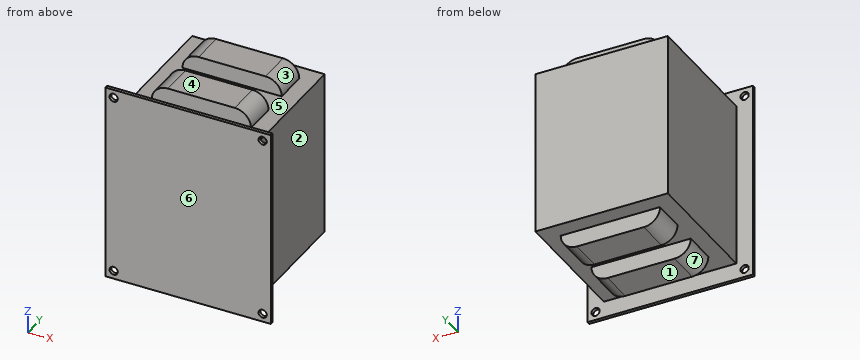
from build123d import *

# Parameters (mm, degrees)
SKETCH1_W           = 127
SKETCH1_H           = 152.4
SKETCH1_R           = 3.175
SKETCH1_W_2         = 101.6
SKETCH1_H_2         = 127
BOSS_EXTRUDE1_DEPTH = 2.54
SKETCH1_4_W         = 101.6
SKETCH1_4_H         = 127
BOSS_EXTRUDE2_DEPTH = 101.6
BOSS_EXTRUDE3_START = 63.5
BOSS_EXTRUDE3_DEPTH = 25.4
BOSS_EXTRUDE4_START = 19.05
BOSS_EXTRUDE4_DEPTH = 25.4


with BuildPart() as part:
    # Sketch1 → Boss-Extrude1 (new body)
    with BuildSketch(Plane(origin=(0, 0, 0), x_dir=(1, 0, 0), z_dir=(0, 1, 0))):
        Rectangle(SKETCH1_W, SKETCH1_H)
        with Locations((-57.15, -69.85)):
            Circle(SKETCH1_R, mode=Mode.SUBTRACT)
        with Locations((57.15, -69.85)):
            Circle(SKETCH1_R, mode=Mode.SUBTRACT)
        with BuildLine():
            Line((-50.8, -63.5), (-50.8, 63.5))
            Line((-50.8, 63.5), (-38.1, 63.5))
            ThreePointArc((-38.1, 63.5), (-34.454650999, 72.300650999), (-25.654, 75.946))
            Line((-25.654, 75.946), (25.654, 75.946))
            ThreePointArc((25.654, 75.946), (34.454650999, 72.300650999), (38.1, 63.5))
            Line((38.1, 63.5), (50.8, 63.5))
            Line((50.8, 63.5), (50.8, -63.5))
            Line((50.8, -63.5), (38.1, -63.5))
            ThreePointArc((38.1, -63.5), (34.454650999, -72.300650999), (25.654, -75.946))
            Line((25.654, -75.946), (-25.654, -75.946))
            ThreePointArc((-25.654, -75.946), (-34.454650999, -72.300650999), (-38.1, -63.5))
            Line((-38.1, -63.5), (-50.8, -63.5))
        make_face(mode=Mode.SUBTRACT)
        with Locations((-57.15, 69.85)):
            Circle(SKETCH1_R, mode=Mode.SUBTRACT)
        with Locations((57.15, 69.85)):
            Circle(SKETCH1_R, mode=Mode.SUBTRACT)
        with BuildLine():
            Line((38.1, -63.5), (-38.1, -63.5))
            ThreePointArc((-38.1, -63.5), (-34.454650999, -72.300650999), (-25.654, -75.946))
            Line((-25.654, -75.946), (25.654, -75.946))
            ThreePointArc((25.654, -75.946), (34.454650999, -72.300650999), (38.1, -63.5))
        make_face()
        Rectangle(SKETCH1_W_2, SKETCH1_H_2)
        with BuildLine():
            ThreePointArc((-25.654, 75.946), (-34.454650999, 72.300650999), (-38.1, 63.5))
            Line((-38.1, 63.5), (38.1, 63.5))
            ThreePointArc((38.1, 63.5), (34.454650999, 72.300650999), (25.654, 75.946))
            Line((25.654, 75.946), (-25.654, 75.946))
        make_face()
    extrude(amount=BOSS_EXTRUDE1_DEPTH)

    # Sketch1<4> → Boss-Extrude2 (add)
    with BuildSketch(Plane(origin=(0, 0, 0), x_dir=(1, 0, 0), z_dir=(0, 1, 0))):
        Rectangle(SKETCH1_4_W, SKETCH1_4_H)
    extrude(amount=BOSS_EXTRUDE2_DEPTH)

    # Sketch1<5> → Boss-Extrude3 (add)
    with BuildSketch(Plane(origin=(0, 0, 0), x_dir=(1, 0, 0), z_dir=(0, 1, 0)).offset(BOSS_EXTRUDE3_START)):
        with BuildLine():
            Line((38.1, -63.5), (-38.1, -63.5))
            ThreePointArc((-38.1, -63.5), (-34.454650999, -72.300650999), (-25.654, -75.946))
            Line((-25.654, -75.946), (25.654, -75.946))
            ThreePointArc((25.654, -75.946), (34.454650999, -72.300650999), (38.1, -63.5))
        make_face()
        with BuildLine():
            Line((25.654, 75.946), (-25.654, 75.946))
            ThreePointArc((-25.654, 75.946), (-34.454650999, 72.300650999), (-38.1, 63.5))
            Line((-38.1, 63.5), (38.1, 63.5))
            ThreePointArc((38.1, 63.5), (34.454650999, 72.300650999), (25.654, 75.946))
        make_face()
    extrude(amount=BOSS_EXTRUDE3_DEPTH)

    # Sketch1<6> → Boss-Extrude4 (add)
    with BuildSketch(Plane(origin=(0, 0, 0), x_dir=(1, 0, 0), z_dir=(0, 1, 0)).offset(BOSS_EXTRUDE4_START)):
        with BuildLine():
            Line((38.1, -63.5), (-38.1, -63.5))
            ThreePointArc((-38.1, -63.5), (-34.454650999, -72.300650999), (-25.654, -75.946))
            Line((-25.654, -75.946), (25.654, -75.946))
            ThreePointArc((25.654, -75.946), (34.454650999, -72.300650999), (38.1, -63.5))
        make_face()
        with BuildLine():
            ThreePointArc((-25.654, 75.946), (-34.454650999, 72.300650999), (-38.1, 63.5))
            Line((-38.1, 63.5), (38.1, 63.5))
            ThreePointArc((38.1, 63.5), (34.454650999, 72.300650999), (25.654, 75.946))
            Line((25.654, 75.946), (-25.654, 75.946))
        make_face()
    extrude(amount=BOSS_EXTRUDE4_DEPTH)


solid = part.part
Model file for the job. Use its own axes, mm. Face numbers are marked on the shaded views. A direction names the side the tool comes from. Give positions to 0.01 mm unless a question says otherwise; leave off trailing zeros. Loops run counter-clockwise (first coordinate to the right, second up) from the corner with the lowest first, then second, coordinate; pieces in that order, holes last.
1) Saw through at A-A (x = 57.15). Write the cut outline in (y, z) (3 decimals).
2) Wall check: line 1 (Z direction, x = 57.15, y = 1.3) (3 decimals); line 2 (X direction, y = 1.45, z = -69.85) (3 decimals); line 3 (Y direction, x = -57.5, z = -58.5). Give the ranges that are in metal, low to high.
3) Saw through at B-B (z = -9.5). Write the cut outline in (x, y).
4) Pull direction Y, two halves, no side cores. Call the marked faces 5, 6 and 7: +Y half, -Y half, draft (parallel to the pull), parting line (faces both ways), or undercut.
5) Saw through at D-D (z = 69.85). Write the cut outline in (x, y) (3 decimals).
6) Flat gauge pins, fed straight in: pin 1 Ø13.5 at (x, z) = (10, -73) entering from +Y; pin 2 Ø8 at (y, z) = (87.5, 54.5) entering from -X; pin 3 Ø1 at (y, z) = (78.5, -4.5) entering from +X; pin 4 Ø5 at (x, z) = (-57.15, -69.85) entering from +Y. Where does each tip first touch, or does it go through?
7) Saw through at C-C (y = 84.5). Write the cut outline in (x, z).
8) Tool access for the marked faces 1, 2, 3 and 4: list every direction of +Z, -Z, +X, -X, +Y, -Y with a clear straight run to the whole face (end or side of a thin tool).
Answer block:
1. outline: (0, -76.2) - (2.54, -76.2) - (2.54, -73.025) - (0, -73.025) - close; (0, -66.675) - (2.54, -66.675) - (2.54, 66.675) - (0, 66.675) - close; (0, 73.025) - (2.54, 73.025) - (2.54, 76.2) - (0, 76.2) - close
2. line 1: z = -76.2 to -73.025, -66.675 to 66.675, 73.025 to 76.2
2. line 2: x = -63.5 to -60.325, -53.975 to 53.975, 60.325 to 63.5
2. line 3: y = 0 to 2.54
3. outline: (-63.5, 0) - (63.5, 0) - (63.5, 2.54) - (50.8, 2.54) - (50.8, 101.6) - (-50.8, 101.6) - (-50.8, 2.54) - (-63.5, 2.54) - close
4. face 5: undercut
4. face 6: -Y half
4. face 7: draft
5. outline: (-63.5, 0) - (-60.325, 0) - (-60.325, 2.54) - (-63.5, 2.54) - close; (-53.975, 0) - (53.975, 0) - (53.975, 2.54) - (-53.975, 2.54) - close; (-36.358, 19.05) - (36.358, 19.05) - (36.358, 44.45) - (-36.358, 44.45) - close; (-36.358, 63.5) - (36.358, 63.5) - (36.358, 88.9) - (-36.358, 88.9) - close; (60.325, 0) - (63.5, 0) - (63.5, 2.54) - (60.325, 2.54) - close
6. pin 1: stops at y = 88.9
6. pin 2: stops at x = -50.8
6. pin 3: stops at x = 50.8
6. pin 4: passes through
7. outline: (-50.8, -63.5) - (-38.1, -63.5) arc R12.45 ccw to (-25.65, -75.95) - (25.65, -75.95) arc R12.45 ccw to (38.1, -63.5) - (50.8, -63.5) - (50.8, 63.5) - (38.1, 63.5) arc R12.45 ccw to (25.65, 75.95) - (-25.65, 75.95) arc R12.45 ccw to (-38.1, 63.5) - (-50.8, 63.5) - close
8. face 1: -Z, +X, -X, +Y
8. face 2: +Z, -Z, +X, +Y
8. face 3: +Z, +X, +Y
8. face 4: +Z, +X, -X, +Y
